Design review of the part built by this model. Coordinates are the model's own, in mm. Give positions to 0.01 mm unless a question says otherwise; leave off trailing zeros. Loops run counter-clockwise (first coordinate to the right, second up) from the corner with the lowest first, then second, coordinate; pieces in that order, holes last. Notation, with made-up numbers: M 39.5,36 L 60.5,36 A14 ccw 60.5,48 Z; hole C -30,51.5 d11. An arc over 180 degrees is marked long. Use a Markdown table: item, result. Add a question column.
(1) Add section A-A, the plane x = 0. Give the boundary of the cut face in (y, z), then the cut area to 3 significant figures.
(2) Insertion check: pin 1 Ø1.5 at (x, z) = (-3, 32) entering from -Y. The pin has a flat end and moves straight along its axis. Give the tip position at first contact, or say it passes through.
(3) For probe 1 along X at (y, z) = (9.5, 30); probe 2 along Z at (x, y) = (-2, 4.5); probe 3 along Z at (x, y) = (1.5, 1.25), list the stretches that pass through material, from the lowest coordinate up.
(4) Add section B-B, the plane y = 6. Give the boundary of the cut face in (x, z).
```python
from build123d import *

# Parameters (mm, degrees)
SKETCH1_W           = 20
SKETCH1_H           = 100
BOSS_EXTRUDE1_DEPTH = 10
CUT_EXTRUDE1_DEPTH  = 10


with BuildPart() as part:
    # Sketch1 → Boss-Extrude1 (new body)
    with BuildSketch(Plane(origin=(0, 0, 0), x_dir=(1, 0, 0), z_dir=(0, 1, 0))):
        Rectangle(SKETCH1_W, SKETCH1_H)
    extrude(amount=BOSS_EXTRUDE1_DEPTH)

    # Sketch2 → Cut-Extrude1 (cut)
    with BuildSketch(Plane(origin=(0, 10, 0), x_dir=(1, 0, 0), z_dir=(0, 1, 0))):
        with BuildLine():
            Line((3.05, 30), (3.05, 20))
            ThreePointArc((3.05, 20), (0, 16.95), (-3.05, 20))
            Line((-3.05, 20), (-3.05, 30))
            ThreePointArc((-3.05, 30), (0, 33.05), (3.05, 30))
        make_face()
    cut_extrude1 = extrude(amount=-CUT_EXTRUDE1_DEPTH, mode=Mode.SUBTRACT)

    # Mirror1: Cut-Extrude1 across plane
    add(cut_extrude1.mirror(Plane.XY), mode=Mode.SUBTRACT)


solid = part.part
```
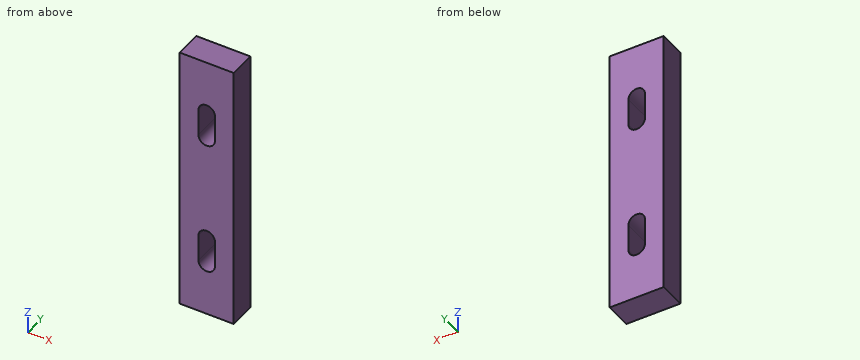
Established:
| question | item | result |
|---|---|---|
| 1 | outline | M 0,-50 L 10,-50 L 10,-33.05 L 0,-33.05 Z; M 0,-16.95 L 10,-16.95 L 10,16.95 L 0,16.95 Z; M 0,33.05 L 10,33.05 L 10,50 L 0,50 Z |
| 1 | area | 678 mm^2 |
| 2 | pin 1 | y = 0 |
| 3 | probe 1 | -10 to -3.05, 3.05 to 10 |
| 3 | probe 2 | -50 to -32.3, -17.7 to 17.7, 32.3 to 50 |
| 3 | probe 3 | -50 to -32.66, -17.34 to 17.34, 32.66 to 50 |
| 4 | outline | M -10,-50 L 10,-50 L 10,50 L -10,50 Z; hole M -3.05,-30 A3.05 ccw 3.05,-30 L 3.05,-20 A3.05 ccw -3.05,-20 Z; hole M -3.05,20 A3.05 ccw 3.05,20 L 3.05,30 A3.05 ccw -3.05,30 Z |
